CAD build for the part. Positions are in the model's coordinates, mm. Face numbers are marked on the shaded views. A direction names the side the tool comes from. Coordinates: 2 decimals unless noted, no trailing zeros. Order: outer loops, then holes, each group sorted by start corner. A loop starts at its lowest first (then second) coordinate and runs counter-clockwise, first axis right, second up. Notation, with made-up numbers: (21, 80) - (74, 80) arc R30 ccw to (74, 106) - close; hole circle Ø9 at (32, 0.5). An arc over 180 degrees is marked (long way). Use one line per item in the form item = value.
```python
from build123d import *

# Parameters (mm, degrees)
SKETCH1_R           = 12.7
BOSS_EXTRUDE1_DEPTH = 6.35
SKETCH2_R           = 11.811
CUT_EXTRUDE1_DEPTH  = 4.7625
SKETCH3_R           = 3.0988
BOSS_EXTRUDE2_DEPTH = 11.43
FILLET1_R           = 1.27


with BuildPart() as part:
    # Sketch1 → Boss-Extrude1 (new body)
    with BuildSketch(Plane(origin=(0, 0, 0), x_dir=(1, 0, 0), z_dir=(0, 1, 0))):
        with Locations(Location((0, 0, 0), (0, 0, 270))):
            Circle(SKETCH1_R)
    extrude(amount=BOSS_EXTRUDE1_DEPTH)

    # Sketch2 → Cut-Extrude1 (cut)
    with BuildSketch(Plane(origin=(0, 6.35, 0), x_dir=(1, 0, 0), z_dir=(0, 1, 0))):
        with Locations(Location((0, 0, 0), (0, 0, 270))):
            Circle(SKETCH2_R)
    extrude(amount=-CUT_EXTRUDE1_DEPTH, mode=Mode.SUBTRACT)

    # Sketch3 → Boss-Extrude2 (add)
    with BuildSketch(Plane.XZ):
        with Locations(Location((0, 0, 0), (0, 0, 270))):
            Circle(SKETCH3_R)
    extrude(amount=BOSS_EXTRUDE2_DEPTH)

    # Fillet1
    fillet1_edges = [part.edges().sort_by_distance(p)[0] for p in [
        (0, -11.43, 3.0988),
        (0, 0, -12.7),
        (0, 0, 3.0988),
    ]]
    fillet(fillet1_edges, radius=FILLET1_R)


solid = part.part
```
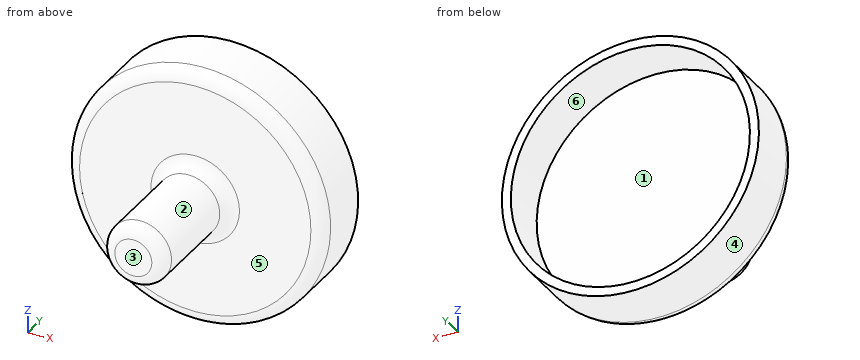
Item 1: Two-plate mould, pull along Z, no slides. Class the marked faces 1, 2 and 3: +Z half, -Z half, draft (parallel to the pull), parting line (faces both ways), or undercut.
Derived:
face_1 = undercut
face_2 = parting line
face_3 = draft
Item 2: Cut at A-A, the plane z = 0. Write the cut outline in (x, y), plus the area to 3 significant figures.
Derived:
outline = (-12.7, 1.27) arc R1.27 ccw to (-11.43, 0) - (-4.37, 0) arc R1.27 cw to (-3.1, -1.27) - (-3.1, -10.16) arc R1.27 ccw to (-1.83, -11.43) - (1.83, -11.43) arc R1.27 ccw to (3.1, -10.16) - (3.1, -1.27) arc R1.27 cw to (4.37, 0) - (11.43, 0) arc R1.27 ccw to (12.7, 1.27) - (12.7, 6.35) - (11.81, 6.35) - (11.81, 1.59) - (-11.81, 1.59) - (-11.81, 6.35) - (-12.7, 6.35) - close
area = 119 mm²
Item 3: 3-axis set-ups, long thin cutter, end or side, ignore diameter. For the marked faces 4, 5 and 6: which of +Z, -Z, +X, -X, +Y, -Y reach the whole face in a straight line?
Derived:
face_4 = +Y, -Y
face_5 = -Y
face_6 = +Y
Item 4: Drop flat-ended pins along their axis: pin 1 (8 mm diameter, centred on y = -7.5, z = 1.5, fed in from -X); pin 2 (7 mm diameter, centred on x = 5, z = 3, fed in from +Y); pin 3 (8 mm diameter, centred on y = -5, z = 7.5, fed in from +X); pin 4 (5 mm diameter, centred on x = 3, y = -2, fed in from -Z). Give the stop position or say it passes through.
Derived:
pin_1 = -3.1
pin_2 = 1.59
pin_3 = through
pin_4 = -12.15
Item 5: Drill centre lines: line 1 (Y direction, x = 10, z = 0.25); line 2 (Y direction, x = 0.5, z = -1.25); line 3 (X direction, y = 3.6, z = 0). Where is each one in solid material? Low to high. Write a range as [from, to].
Derived:
line_1 = [0, 1.59]
line_2 = [-11.43, 1.59]
line_3 = [-12.7, -11.81], [11.81, 12.7]
Item 6: Cut at B-B, the plane x = 0. Write the cut outline in (y, z).
Derived:
outline = (-11.43, -1.83) arc R1.27 ccw to (-10.16, -3.1) - (-1.27, -3.1) arc R1.27 cw to (0, -4.37) - (0, -11.43) arc R1.27 ccw to (1.27, -12.7) - (6.35, -12.7) - (6.35, -11.81) - (1.59, -11.81) - (1.59, 11.81) - (6.35, 11.81) - (6.35, 12.7) - (1.27, 12.7) arc R1.27 ccw to (0, 11.43) - (0, 4.37) arc R1.27 cw to (-1.27, 3.1) - (-10.16, 3.1) arc R1.27 ccw to (-11.43, 1.83) - close
Item 7: Cut at C-C, the plane y = -3. Write the cut outline in (x, z), plus the area to 3 significant figures.
Derived:
outline = circle Ø6.2 at (0, 0)
area = 30.2 mm²
